Here's how the part is built. I have some questions about the finished solid (model axes, mm). A direction names the side the tool comes from. Coordinates: 2 decimals unless noted, no trailing zeros. Order: outer loops, then holes, each group sorted by start corner. A loop starts at its lowest first (then second) coordinate and runs counter-clockwise, first axis right, second up. Notation, with made-up numbers: (-35.75, -32) - (-23.75, -32) arc R25 ccw to (-23.75, -6) - close; hole circle Ø5 at (0, -25.5). An arc over 180 degrees is marked (long way). Answer in a Markdown table with one row per item. Add a question column.
Item 1: Thinking about a two-plate mould opening in X: for faces 6 (the flat face through (-18, -3, 17)), 7 (the flat face through (-19, -4, -25)), 8 (the flat face through (-9, -4, 17)), which applies, +X half, -X half, draft (parallel to the pull), parting line (faces both ways), or undercut?
Item 2: On a 3-axis mill with a long thin cutter (end or side, diameter ignored), from which of +Z, -Z, +X, -X, +Y, -Y can I reach the whole of each face in a straight line? I mean faces 1 (the flat face through (-3, -2, -12)), 2 (the flat face through (7, -7, 0)), 3 (the flat face through (-18, -3, 0)), 4 (the flat face through (-11, 0, 2)), 5 (the cylindrical face through (-23.75, -5, 12.56)). Say none if no direction works.
Item 3: I want a section at A-A (x = -18). Please give me the cut outline in (y, z).
Item 4: I want a section at B-B (z = 7.5). Please give me the cut outline in (x, y), plus the area to 3 significant figures.
Item 5: I want a section at D-D (x = -13). Please give me the cut outline in (y, z).
Item 6: I want a section at C-C (x = 0). Please give me the cut outline in (y, z).
Item 7: Will these pins go through, and if not, where does the flat tip stop? pin 1 Ø4.5 at (x, y) = (-3, -3.5) entering from -Z; pin 2 Ø2 at (y, z) = (2, -3) entering from +X; pin 3 Ø3.5 at (x, y) = (0, 0) entering from +Z; pin 4 Ø2 at (x, y) = (-2.5, -4.5) entering from +Z.
Item 8: If I drill on line 1 along Y through (x, z) = (0, 7); line 2 along Z through (x, y) = (-8.5, -3.75); line 3 along X through (y, z) = (-5.75, -16), over which ranges is the centre line in solid material (lowest first)? Write a range as from..to.
```python
from build123d import *

# Parameters (mm, degrees)
BOSS_EXTRUDE1_DEPTH = 25
MOUNT_HOLES_DEPTH   = 41.422765863
SKETCH7_W           = 16.5
SKETCH7_H           = 13
CUT_PART_DEPTH      = 20
SKETCH10_R          = 2.75
CUT_EXTRUDE3_DEPTH  = 25
CHAMFER1_SIZE       = 2
CUT_EXTRUDE4_DEPTH  = 3
CHAMFER2_SIZE       = 3


with BuildPart() as part:
    # contour → Boss-Extrude1 (new, symmetric)
    with BuildSketch(Plane.XY):
        with BuildLine():
            Line((0, -7.5), (6.5, -7.5))
            Line((6.5, -7.5), (7.5, -6.5))
            Line((7.5, -6.5), (7.5, 0))
            ThreePointArc((7.5, 0), (-3.9135e-05, 7.5), (-7.5, -7.827e-05))
            Line((-7.5, -7.827e-05), (-28, -7.827e-05))
            Line((-28, -7.827e-05), (-28, -7.5))
            Line((-28, -7.5), (0, -7.5))
        make_face()
    extrude(amount=BOSS_EXTRUDE1_DEPTH, both=True)

    # Sketch6 → mount-holes (cut, through all)
    with BuildSketch(Plane.XZ.offset(7.5)):
        with BuildLine():
            Line((-21, 15.25), (-17, 15.25))
            ThreePointArc((-17, 15.25), (-14.25, 12.5), (-17, 9.75))
            Line((-17, 9.75), (-21, 9.75))
            ThreePointArc((-21, 9.75), (-23.75, 12.5), (-21, 15.25))
        make_face()
        with BuildLine():
            Line((-21, -9.75), (-17, -9.75))
            ThreePointArc((-17, -9.75), (-14.25, -12.5), (-17, -15.25))
            Line((-17, -15.25), (-21, -15.25))
            ThreePointArc((-21, -15.25), (-23.75, -12.5), (-21, -9.75))
        make_face()
    extrude(amount=-MOUNT_HOLES_DEPTH, mode=Mode.SUBTRACT)

    # Sketch7 → cut-part (cut)
    with BuildSketch(Plane.XZ.offset(7.5)):
        with Locations((-0.75, 18.5)):
            Rectangle(SKETCH7_W, SKETCH7_H)
        with Locations((-0.75, -18.5)):
            Rectangle(SKETCH7_W, SKETCH7_H)
    extrude(amount=-CUT_PART_DEPTH, mode=Mode.SUBTRACT)

    # Sketch10 → Cut-Extrude3 (cut, symmetric)
    with BuildSketch(Plane.XY):
        Circle(SKETCH10_R)
    extrude(amount=CUT_EXTRUDE3_DEPTH, both=True, mode=Mode.SUBTRACT)

    # Chamfer1
    chamfer1_edges = [part.edges().sort_by_distance(p)[0] for p in [
        (-28, -3.750039135, 25),
        (-9, -3.750039135, 25),
        (-28, -3.750039135, -25),
        (-9, -3.750039135, -25),
    ]]
    chamfer(chamfer1_edges, length=CHAMFER1_SIZE)

    # Sketch11 → Cut-Extrude4 (cut)
    with BuildSketch(Plane(origin=(0, -7.827e-05, 0), x_dir=(1, 0, 0), z_dir=(0, 1, 0))):
        Polygon((-11.5, -21.757359313), (-11.5, 21.757359313), (-11.742640687, 22), (-24.757359313, 22), (-25, 21.757359313), (-25, -21.757359313), (-24.757359313, -22), (-11.742640687, -22), align=None)
    extrude(amount=-CUT_EXTRUDE4_DEPTH, mode=Mode.SUBTRACT)

    # Chamfer2
    # the kernel refuses this chamfer: 3 mm, written as the material it adds along each edge
    with BuildSketch(Plane(origin=(-11.5, -3.00007827, 29.472408277), x_dir=(0.027495876610585626, 0.9996219169112968, 0), z_dir=(0, 0, -1))) as chamfer2_piece_1_section:
        Polygon((CHAMFER2_SIZE * 0.999621916911, -CHAMFER2_SIZE * 0.0274958766106), (-CHAMFER2_SIZE * 0.0274958766106, -CHAMFER2_SIZE * 0.999621916911), (0, 0), align=None)
    chamfer2_piece_1 = extrude(amount=58.944816554, mode=Mode.PRIVATE)
    chamfer2_piece_1 = split(chamfer2_piece_1, bisect_by=Plane(origin=(-12.500072931, -2.000114735, -22), z_dir=(0, 0, 1)), keep=Keep.TOP, mode=Mode.PRIVATE)
    chamfer2_piece_1 = split(chamfer2_piece_1, bisect_by=Plane(origin=(-1.121356809, -2.000114735, 11.378716122), z_dir=(-0.7071067811865476, 0, -0.7071067811865476)), keep=Keep.TOP, mode=Mode.PRIVATE)
    chamfer2_piece_1 = chamfer2_piece_1 - Plane(origin=(-17, -2.000114735, -12.5), x_dir=(0, 0, 1), z_dir=(0, -1, 0)) * Cylinder(2.75, 130, mode=Mode.PRIVATE)
    chamfer2_piece_1 = chamfer2_piece_1 - Plane(origin=(-17, -2.000114735, 12.5), x_dir=(0, 0, 1), z_dir=(0, -1, 0)) * Cylinder(2.75, 130, mode=Mode.PRIVATE)
    add(chamfer2_piece_1)
    with BuildSketch(Plane(origin=(-32.472408277, -3.00007827, 22), x_dir=(0, 0.9996219169112968, 0.027495876610586778), z_dir=(1, 0, 0))) as chamfer2_piece_2_section:
        Polygon((CHAMFER2_SIZE * 0.999621916911, -CHAMFER2_SIZE * 0.0274958766106), (-CHAMFER2_SIZE * 0.0274958766106, -CHAMFER2_SIZE * 0.999621916911), (0, 0), align=None)
    chamfer2_piece_2 = extrude(amount=28.444816553, mode=Mode.PRIVATE)
    chamfer2_piece_2 = split(chamfer2_piece_2, bisect_by=Plane(origin=(-11.5, -2.001383642, 20.997389255), z_dir=(-1, 0, 0)), keep=Keep.TOP, mode=Mode.PRIVATE)
    chamfer2_piece_2 = split(chamfer2_piece_2, bisect_by=Plane(origin=(-22.004985029, -2.001383642, 24.752374284), z_dir=(0.7071067811865527, 0, -0.7071067811865424)), keep=Keep.TOP, mode=Mode.PRIVATE)
    add(chamfer2_piece_2)
    with BuildSketch(Plane(origin=(-25, -3.00007827, -29.472408277), x_dir=(-0.027495876610586778, 0.9996219169112968, 0), z_dir=(0, 0, 1))) as chamfer2_piece_3_section:
        Polygon((CHAMFER2_SIZE * 0.999621916911, -CHAMFER2_SIZE * 0.0274958766106), (-CHAMFER2_SIZE * 0.0274958766106, -CHAMFER2_SIZE * 0.999621916911), (0, 0), align=None)
    chamfer2_piece_3 = extrude(amount=58.944816554, mode=Mode.PRIVATE)
    chamfer2_piece_3 = split(chamfer2_piece_3, bisect_by=Plane(origin=(-35.402787978, -1.975969948, -11.354571334), z_dir=(0.7071067811865527, 0, 0.7071067811865424)), keep=Keep.TOP, mode=Mode.PRIVATE)
    chamfer2_piece_3 = split(chamfer2_piece_3, bisect_by=Plane(origin=(-24.048216644, -1.975969948, 22), z_dir=(0, 0, -1)), keep=Keep.TOP, mode=Mode.PRIVATE)
    chamfer2_piece_3 = chamfer2_piece_3 - Plane(origin=(-21, -1.975969948, -12.5), x_dir=(0, 0, -1), z_dir=(0, -1, 0)) * Cylinder(2.75, 130, mode=Mode.PRIVATE)
    chamfer2_piece_3 = chamfer2_piece_3 - Plane(origin=(-21, -1.975969948, 12.5), x_dir=(0, 0, -1), z_dir=(0, -1, 0)) * Cylinder(2.75, 130, mode=Mode.PRIVATE)
    add(chamfer2_piece_3)
    with BuildSketch(Plane(origin=(-4.027591723, -3.00007827, -22), x_dir=(0, 0.9996219169112968, -0.027495876610586778), z_dir=(-1, 0, 0))) as chamfer2_piece_4_section:
        Polygon((CHAMFER2_SIZE * 0.999621916911, -CHAMFER2_SIZE * 0.0274958766106), (-CHAMFER2_SIZE * 0.0274958766106, -CHAMFER2_SIZE * 0.999621916911), (0, 0), align=None)
    chamfer2_piece_4 = extrude(amount=28.444816553, mode=Mode.PRIVATE)
    chamfer2_piece_4 = split(chamfer2_piece_4, bisect_by=Plane(origin=(-11.5, -2.001383642, -20.997389255), z_dir=(-1, 0, 0)), keep=Keep.TOP, mode=Mode.PRIVATE)
    chamfer2_piece_4 = split(chamfer2_piece_4, bisect_by=Plane(origin=(-25, -2.001383642, -20.997389255), z_dir=(1, 0, 0)), keep=Keep.TOP, mode=Mode.PRIVATE)
    add(chamfer2_piece_4)


solid = part.part
```
Values follow:
| question | item | result |
|---|---|---|
| 1 | face 6 | undercut |
| 1 | face 7 | draft |
| 1 | face 8 | +X half |
| 2 | face 1 | -Z, +X, +Y, -Y |
| 2 | face 2 | +Z, -Z, +X, -Y |
| 2 | face 3 | +Y |
| 2 | face 4 | +Z, -Z, -X, +Y |
| 2 | face 5 | +Y, -Y |
| 3 | outline | (-7.5, -25) - (0, -25) - (0, -22) - (-3, -19) - (-3, -15.25) - (-7.5, -15.25) - close; (-7.5, -9.75) - (-3, -9.75) - (-3, 9.75) - (-7.5, 9.75) - close; (-7.5, 15.25) - (-3, 15.25) - (-3, 19) - (0, 22) - (0, 25) - (-7.5, 25) - close |
| 4 | outline | (-28, -7.5) - (6.5, -7.5) - (7.5, -6.5) - (7.5, 0) arc R7.5 ccw to (-7.5, 0) - (-11.5, 0) - (-14.5, -3) - (-22, -3) - (-25, 0) - (-28, 0) - close; hole circle Ø5.5 at (0, 0) |
| 4 | area | 299 mm^2 |
| 5 | outline | (-7.5, -25) - (0, -25) - (0, -22) - (-1.5, -20.5) - (-1.5, 20.5) - (0, 22) - (0, 25) - (-7.5, 25) - close |
| 6 | outline | (-7.5, -12) - (-2.75, -12) - (-2.75, 12) - (-7.5, 12) - close; (2.75, -12) - (7.5, -12) - (7.5, 12) - (2.75, 12) - close |
| 7 | pin 1 | stops at z = -12 |
| 7 | pin 2 | stops at x = 7.43 |
| 7 | pin 3 | passes through |
| 7 | pin 4 | stops at z = 12 |
| 8 | line 1 | y = -7.5..-2.75, 2.75..7.5 |
| 8 | line 2 | z = -12..12 |
| 8 | line 3 | x = -28..-9 |
